from build123d import *

# Parameters (mm, degrees)
F1_DEPTH = 381
F2_R     = 12.7
F3_DEPTH = 381
F5_R     = 12.7
F6_DEPTH = 25.4
F4_R     = 12.7
F7_DEPTH = 25.4


with BuildPart() as f1:
    # F0 (on Front) → F1 (new body)
    with BuildSketch(Plane.XZ):
        Polygon((-99.244288, 21.165265), (-231.226559, -55.034735), (149.773441, -55.034735), (281.755712, 21.165265), align=None)
    extrude(amount=F1_DEPTH)

    # F2 (on face) → F3 (cut)
    with BuildSketch(Plane.XZ.offset(381)):
        with Locations((25.264577, -16.934735)):
            Circle(F2_R)
    extrude(amount=-F3_DEPTH, mode=Mode.SUBTRACT)

    # F5 (on face) → F6 (cut)
    with BuildSketch(Plane(origin=(0, 0, -55.034735), x_dir=(1, 0, 0), z_dir=(0, 0, -1))):
        with Locations((-40.726559, 190.5)):
            Circle(F5_R)
    extrude(amount=-F6_DEPTH, mode=Mode.SUBTRACT)

    # F4 (on face) → F7 (cut)
    with BuildSketch(Plane.XY.offset(21.165265)):
        with Locations((91.255712, -190.5)):
            Circle(F4_R)
    extrude(amount=-F7_DEPTH, mode=Mode.SUBTRACT)


solid = f1.part
Model file for the job. Use its own axes, mm. A direction names the side the tool comes from. Give positions to 0.01 mm unless a question says otherwise; leave off trailing zeros. Write each loop counter-clockwise with the first axis right and the second up, starting at its lowest first coordinate (ties: lowest second). Pieces come first, ordered by that corner, then holes. Notation, with made-up numbers: M -19.5,-19 L -1.5,-19 A12 cw -1.5,-4 Z; hole C 55,-30.75 d1. An arc over 180 degrees is marked long. One line per item, written item: value. Start each with the question number.
Q1. Saw through at D-D, the plane x = 200.5. Write the cut outline in (y, z), plus the area to 3 significant figures.
Q2. Two-plate mould, pull along Y, no slides. Class faces 1 (the cylindrical face through (89, -203, 9)), 2 (the flat face through (-43, -145, -55.035)), 3 (the flat face through (22, 0, -33)), 4 (the flat face through (22, -381, -33)): +Y half, -Y half, draft (parallel to the pull), parting line (faces both ways), or undercut.
Q3. Saw through at B-B, the plane z = -11. Write the cut outline in (x, y), plus the area to 3 significant figures.
Q4. Drop flat-ended pins along their axis: pin 1 Ø1.5 at (y, z) = (-334, -45) entering from -X; pin 2 Ø15 at (x, z) = (25.26, -16.93) entering from -Y; pin 3 Ø4 at (y, z) = (-292.5, -45) entering from -X; pin 4 Ø3 at (y, z) = (-189, 5) entering from -X. Give the stop position or say it passes through.
Q5. Saw through at C-C, the plane z = -40. Write the cut outline in (x, y), plus the area to 3 significant figures.
Q6. 3-axis set-ups, long thin cutter, end or side, ignore diameter. For faces 5 (the cylindrical face through (-43.48, -178.102, -42.513)), 6 (the flat face through (214.84, -187.83, -17.47)), 7 (the flat face through (91, -190, -4.235)): which of +Z, -Z, +X, -X, +Y, -Y reach the whole face in a straight line?
Q7. Saw through at A-A, the plane y = -190.5. Write the cut outline in (x, z), plus the area to 3 significant figures.
Q8. Probe probe 1 along X at (y, z) = (-35, -17); probe 2 along X at (y, z) = (-290.5, -26.5); probe 3 along Z at (x, y) = (-135, -295.5). List the from-to ranges inside material, lowest first. Write a range as [from, to].
Output values:
1. outline: M -381,-25.75 L 0,-25.75 L 0,21.17 L -381,21.17 Z
1. area: 17,900 mm²
2. face 1: undercut
2. face 2: draft
2. face 3: +Y half
2. face 4: -Y half
3. outline: M -154.96,-381 L 14.04,-381 L 14.04,0 L -154.96,0 Z; M 36.49,-381 L 226.04,-381 L 226.04,0 L 36.49,0 Z
3. area: 137,000 mm²
4. pin 1: stops at x = -215.14
4. pin 2: passes through
4. pin 3: stops at x = -217.31
4. pin 4: stops at x = -129.84
5. outline: M -205.19,-381 L 175.81,-381 L 175.81,0 L -205.19,0 Z; hole C -40.73,-190.5 d25.4
5. area: 145,000 mm²
6. face 5: -Z
6. face 6: -Z, +X, +Y, -Y
6. face 7: +Z
7. outline: M -231.23,-55.03 L -53.43,-55.03 L -53.43,-29.63 L -28.03,-29.63 L -28.03,-55.03 L 149.77,-55.03 L 281.76,21.17 L 103.96,21.17 L 103.96,-4.23 L 78.56,-4.23 L 78.56,21.17 L -99.24,21.17 Z; hole C 25.26,-16.93 d25.4
7. area: 27,200 mm²
8. probe 1: x = [-165.35, 12.56], [37.96, 215.65]
8. probe 2: x = [-181.8, 16.91], [33.62, 199.2]
8. probe 3: z = [-55.03, 0.52]
